CAD build for the part. Positions are in the model's coordinates, mm. Coordinates: 2 decimals unless noted, no trailing zeros. Loops run counter-clockwise (first coordinate to the right, second up) from the corner with the lowest first, then second, coordinate; pieces in that order, holes last. Notation, with made-up numbers: (29.5, 25) -> (52.5, 25) arc R27 ccw to (52.5, 63) -> close; hole circle Ø6 at (79, -4.5). An arc over 180 degrees is marked (long way). Write each question's results on one line, items separated by ' | '.
from build123d import *

# Parameters (mm, degrees)
F0_W     = 10
F0_H     = 25
F0_R     = 1.6
F1_DEPTH = 10
F2_R     = 3
F3_SIZE  = 1.5


with BuildPart() as f1:
    # F0 (on Top) → F1 (new body)
    with BuildSketch(Plane.XY):
        Rectangle(F0_W, F0_H)
        with Locations((0, -7.5)):
            Circle(F0_R, mode=Mode.SUBTRACT)
        with Locations((0, 7.5)):
            Circle(F0_R, mode=Mode.SUBTRACT)
    extrude(amount=F1_DEPTH)

    # F2
    f2_edges = [f1.edges().sort_by_distance(p)[0] for p in [
        (-5, 12.5, 5),
        (-5, -12.5, 5),
        (5, -12.5, 5),
        (5, 12.5, 5),
    ]]
    fillet(f2_edges, radius=F2_R)

    # F3
    f3_edges = [f1.edges().sort_by_distance(p)[0] for p in [
        (-1.6, 7.5, 10),
        (-1.6, -7.5, 10),
    ]]
    chamfer(f3_edges, length=F3_SIZE)


solid = f1.part
1) Slice it at C-C (y = 7.5). Write the cut outline in (x, z), then the cut area to 4 significant figures.
Outcome:
outline: (-5, 0) -> (-1.6, 0) -> (-1.6, 8.5) -> (-3.1, 10) -> (-5, 10) -> close; (1.6, 0) -> (5, 0) -> (5, 10) -> (3.1, 10) -> (1.6, 8.5) -> close | area: 65.75 mm^2
2) Pin check, flat tips, straight feed: pin 1 (1 mm diameter, centred on x = -1, y = 6, fed in from +Z); pin 2 (3.5 mm diameter, centred on x = 0, y = -7.5, fed in from +Z). Stop position of each tip, or through.
Outcome:
pin 1: stops at z = 9.2 | pin 2: stops at z = 8.65
3) Slice it at B-B (z = 9). Write the cut outline in (x, y).
Outcome:
outline: (-5, -9.5) arc R3 ccw to (-2, -12.5) -> (2, -12.5) arc R3 ccw to (5, -9.5) -> (5, 9.5) arc R3 ccw to (2, 12.5) -> (-2, 12.5) arc R3 ccw to (-5, 9.5) -> close; hole circle Ø4.2 at (0, -7.5); hole circle Ø4.2 at (0, 7.5)
4) Drill centre lines: L1, parallel to Y at x = 0, z = 3; L2, parallel to Y at x = 0.5, z = 1; L3, parallel to X at y = 8, z = 4.5. Where is each one in solid material? Low to high. Write a range as from..to.
Outcome:
L1: y = -12.5..-9.1, -5.9..5.9, 9.1..12.5 | L2: y = -12.5..-9.02, -5.98..5.98, 9.02..12.5 | L3: x = -5..-1.52, 1.52..5
5) Slice it at A-A (x = 0). Write the cut outline in (y, z), then the cut area to 4 significant figures.
Outcome:
outline: (-12.5, 0) -> (-9.1, 0) -> (-9.1, 8.5) -> (-10.6, 10) -> (-12.5, 10) -> close; (-5.9, 0) -> (5.9, 0) -> (5.9, 8.5) -> (4.4, 10) -> (-4.4, 10) -> (-5.9, 8.5) -> close; (9.1, 0) -> (12.5, 0) -> (12.5, 10) -> (10.6, 10) -> (9.1, 8.5) -> close | area: 181.5 mm^2
6) Two-plate mould, pull along Y, no slides. Class faces 1 (the cylindrical face through (4.1, 11.64, 5.07)), 2 (the flat face through (5, 0, 5)), 3 (the cylindrical face through (-0.35, 5.94, 4.19)), 4 (the cylindrical face through (4.1, -11.64, 5.07)): pulls with the +Y half, pulls with the -Y half, needs draft (parallel to the pull), parting line crosses it, or undercut.
Outcome:
face 1: pulls with the +Y half | face 2: needs draft | face 3: undercut | face 4: pulls with the -Y half
7) Slice it at D-D (z = 7.25). Write the cut outline in (x, y), then the cut area to 3 significant figures.
Outcome:
outline: (-5, -9.5) arc R3 ccw to (-2, -12.5) -> (2, -12.5) arc R3 ccw to (5, -9.5) -> (5, 9.5) arc R3 ccw to (2, 12.5) -> (-2, 12.5) arc R3 ccw to (-5, 9.5) -> close; hole circle Ø3.2 at (0, -7.5); hole circle Ø3.2 at (0, 7.5) | area: 226 mm^2
